Work out the finished part from the listing and answer in its coordinate system (mm). Face numbers are marked on the shaded views. A direction names the side the tool comes from. Round coordinates to 2 decimals unless told otherwise and drop trailing zeros. Order: outer loops, then holes, each group sorted by start corner. A loop starts at its lowest first (then second) coordinate and runs counter-clockwise, first axis right, second up. Notation, with made-up numbers: M -24,17 L 25,17 A28 cw 25,52 Z; hole C -15.75,87.5 d8. An arc over 180 degrees is marked long. Answer as a JSON object with one key per item and string values. Group by question number.
from build123d import *

# Parameters (mm, degrees)
F0_W     = 35
F0_H     = 57
F1_DEPTH = 25
F2_T     = -1.5
F4_D     = 2


with BuildPart() as f1:
    # F0 (on Top) → F1 (new body)
    with BuildSketch(Plane.XY):
        Rectangle(F0_W, F0_H)
    extrude(amount=F1_DEPTH)

    # F2
    f2_openings = [f1.faces().sort_by_distance(p)[0] for p in [
        (0, 0, 25),
    ]]
    offset(amount=F2_T, openings=f2_openings)

    # F4 (through all)
    with Locations(Plane.XZ.offset(28.5)):
        with Locations((-9.480757, 14.56372), (0, 14.56372)):
            Hole(F4_D / 2)


solid = f1.part
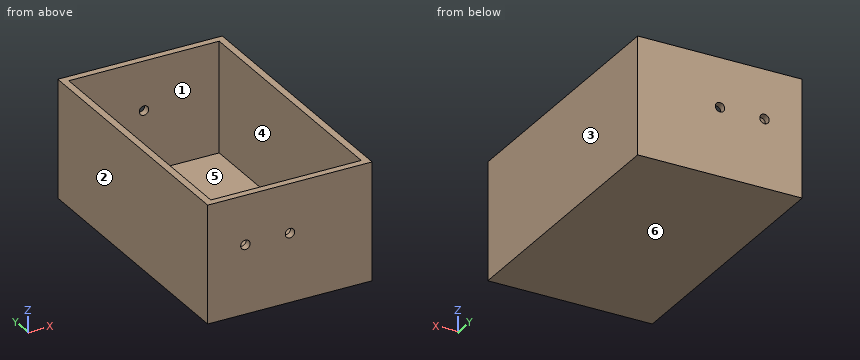
Item 1: Find section D-D (x = 3.5). Give the vertices of the cut face in (y, z), and give its area (3 significant figures).
Item 2: Consider L1, parallel to X at y = -12, z = 1.75; L2, parallel to Z at x = 0, y = -28.1; L3, parallel to Y at x = 7, z = 16.5. Determine where each line is inside the solid, lowest interval first.
Item 3: This flat-tipped pin is pushed along its axis until it touches: pin 1 (9.5 mm diameter, centred on x = -3.5, y = 2, fed in from +Z). Where does it stop, or does it pass through?
Item 4: Find section B-B (x = 0). Give the vertices of the cut face in (y, z), and give its area (3 significant figures).
Item 5: Find section A-A (z = 7.25). Give the vertices of the cut face in (x, y).
Item 6: The mould has two halves that part along X. Classify the marked faces 3, 4, 5 and 6: +X half, -X half, draft (parallel to the pull), parting line (faces both ways), or undercut.
Item 7: A tool of negligible diameter and unlimited length cuts with its end or side. For the marked faces 1 and 2, from which of +Z, -Z, +X, -X, +Y, -Y can it reach the whole face along a straight path? Write none if from no direction.
Item 8: Find section C-C (y = -17.5). Give the vertices of the cut face in (x, z).
Responses:
{
 "1": {"outline": "M -28.5,0 L 28.5,0 L 28.5,25 L 27,25 L 27,1.5 L -27,1.5 L -27,25 L -28.5,25 Z", "area": "156 mm^2"},
 "2": {"L1": "x = -17.5 to -16, 16 to 17.5", "L2": "z = 0 to 13.56, 15.56 to 25", "L3": "y = -28.5 to -27, 27 to 28.5"},
 "3": {"pin 1": "stops at z = 1.5"},
 "4": {"outline": "M -28.5,0 L 28.5,0 L 28.5,13.56 L 27,13.56 L 27,1.5 L -27,1.5 L -27,13.56 L -28.5,13.56 Z; M -28.5,15.56 L -27,15.56 L -27,25 L -28.5,25 Z; M 27,15.56 L 28.5,15.56 L 28.5,25 L 27,25 Z", "area": "150 mm^2"},
 "5": {"outline": "M -17.5,-28.5 L 17.5,-28.5 L 17.5,28.5 L -17.5,28.5 Z; hole M -16,-27 L 16,-27 L 16,27 L -16,27 Z"},
 "6": {"face 3": "+X half", "face 4": "undercut", "face 5": "undercut", "face 6": "draft"},
 "7": {"face 1": "+Z", "face 2": "+Z, -Z, -X, +Y, -Y"},
 "8": {"outline": "M -17.5,0 L 17.5,0 L 17.5,25 L 16,25 L 16,1.5 L -16,1.5 L -16,25 L -17.5,25 Z"}
}
